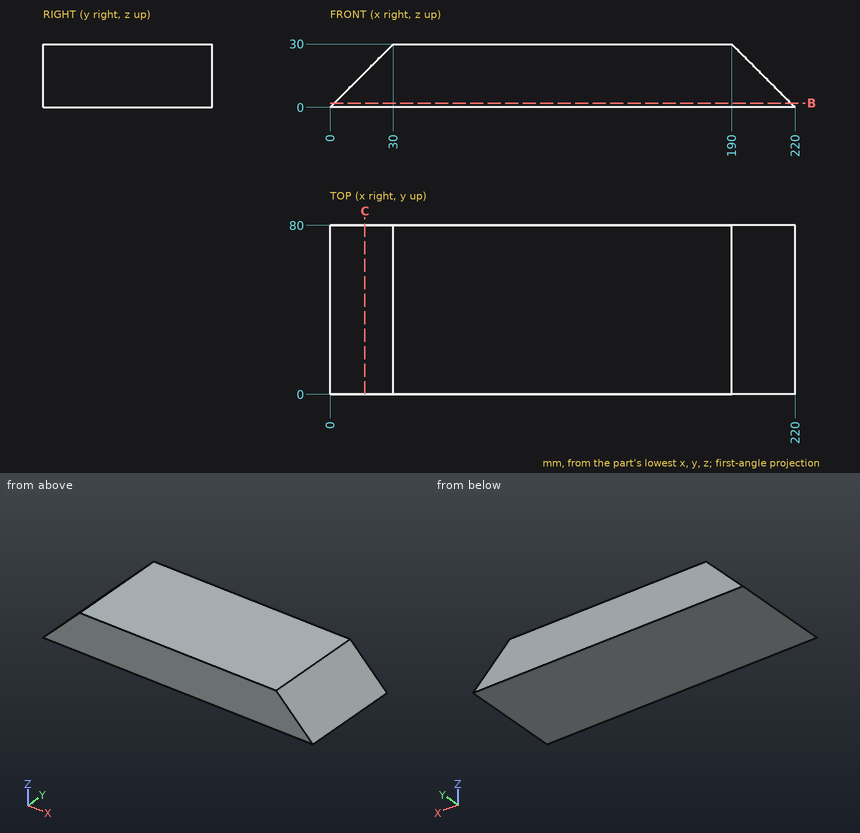
Geometry check sheet. Reference: drawing and pictorial views, mm from the part's lowest x, y, z. Round coordinates to 2 decimals unless told otherwise and drop trailing zeros. Loops run counter-clockwise (first coordinate to the right, second up) from the corner with the lowest first, then second, coordinate; pieces in that order, holes last. Notation, with made-up numbers: (34, 63.25) -> (46, 63.25) arc R28 cw to (46, 81.25) -> close; hole circle Ø7 at (71.25, 5). An arc over 180 degrees is marked (long way). Use a Markdown table: item, result.
(1) Sectioned sample at C-C (x = 16.5). Enter the section's corners in (y, z).
Calculated:
| item | result |
|---|---|
| outline | (0, 0) -> (80, 0) -> (80, 16.5) -> (0, 16.5) -> close |
(2) Sectioned sample at B-B (z = 2). Enter the section's corners in (x, y).
Calculated:
| item | result |
|---|---|
| outline | (2, 0) -> (218, 0) -> (218, 80) -> (2, 80) -> close |
(3) Go/stop test with flat-tipped pins: P1, Ø3, axis at y = 14.5, z = 6, coming from the -X side; P2, Ø3, axis at y = 12, z = 14.5, coming from the -X side; P3, Ø4, axis at y = 21, z = 20.5, coming from the -X side. Record where each tip stops, or that it passes through.
Calculated:
| item | result |
|---|---|
| P1 | x = 4.5 |
| P2 | x = 13 |
| P3 | x = 18.5 |
(4) Scan lines: probe 1 along X at (y, z) = (7.5, 7.75); probe 2 along X at (y, z) = (64.5, 1.5); probe 3 along Z at (x, y) = (13, 32.5). Record each from-to range of solid material in increasing order.
Calculated:
| item | result |
|---|---|
| probe 1 | 7.75 to 212.25 |
| probe 2 | 1.5 to 218.5 |
| probe 3 | 0 to 13 |
